Part print with two shaded views. Sizes in mm from the minimum x, y, z corner. Coordinates: 2 decimals unless noted, no trailing zeros. Loops run counter-clockwise (first coordinate to the right, second up) from the corner with the lowest first, then second, coordinate; pieces in that order, holes last. Notation, with made-up numbers: (20, 38.5) -> (62, 38.5) arc R33 ccw to (62, 74.5) -> close; hole circle Ø1 at (-34.5, 39). An arc over 180 degrees is marked (long way). Write each question's results on one line, items separated by ' | '.
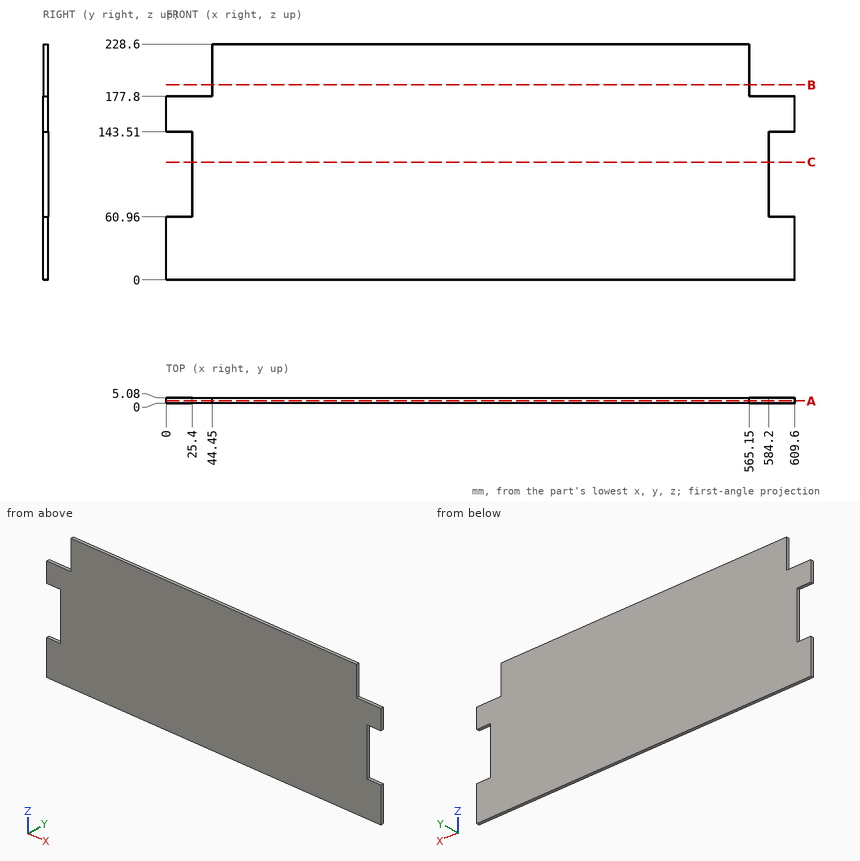
Q1. Drop flat-ended pins along their axis: pin 1 (2.5 mm diameter, centred on y = 2, z = 90, fed in from -X); pin 2 (1 mm diameter, centred on x = 189, z = 135, fed in from -Y); pin 3 (2.5 mm diameter, centred on x = 599, y = 3, fed in from +Z); pin 4 (1.5 mm diameter, centred on y = 3, z = 117.5, fed in from +X). Give the stop position or say it passes through.
Results are:
pin 1: x = 25.4 | pin 2: y = 0 | pin 3: z = 177.8 | pin 4: x = 584.2
Q2. Wall check: L1, parallel to X at y = 4.5, z = 78.5; L2, parallel to X at y = 4.15, z = 217. Give the ranges that are in metal, low to high. Write a range as from..to.
Results are:
L1: 25.4..584.2 | L2: 44.45..565.15
Q3. Cut at B-B on z = 189. Write the cut outline in (x, y).
Results are:
outline: (44.45, 0) -> (565.15, 0) -> (565.15, 5.08) -> (44.45, 5.08) -> close
Q4. Cut at A-A on y = 2.2. Write the cut outline in (x, z), and give its area (3 significant figures).
Results are:
outline: (0, 0) -> (609.6, 0) -> (609.6, 60.96) -> (584.2, 60.96) -> (584.2, 143.51) -> (609.6, 143.51) -> (609.6, 177.8) -> (565.15, 177.8) -> (565.15, 228.6) -> (44.45, 228.6) -> (44.45, 177.8) -> (0, 177.8) -> (0, 143.51) -> (25.4, 143.51) -> (25.4, 60.96) -> (0, 60.96) -> close | area: 131,000 mm^2
Q5. Cut at C-C on z = 114. Write the cut outline in (x, y), and give its area (3 significant figures).
Results are:
outline: (25.4, 0) -> (584.2, 0) -> (584.2, 5.08) -> (25.4, 5.08) -> close | area: 2,840 mm^2
